Verification items for the finished model (mm, model axes). A direction names the side the tool comes from. Give positions to 0.01 mm unless a question says otherwise; leave off trailing zeros. Order: outer loops, then holes, each group sorted by start corner. A loop starts at its lowest first (then second) coordinate and runs counter-clockwise, first axis right, second up. Notation, with made-up numbers: (71, 73.5) - (100, 73.5) arc R22 cw to (100, 105.5) - close; hole circle Ø1 at (44.5, 6.25). An arc over 180 degrees is marked (long way). Answer as a JSON object with one key per item and string values.
```python
from build123d import *

# Parameters (mm, degrees)
F1_DEPTH = 2
F2_R     = 3
F3_R     = 9
F4_W     = 2
F4_H     = 5
F5_DEPTH = 10
F6_R     = 0.99999


# Not quite as in the source:
# - a fillet or chamfer is up to 0.001 mm smaller than in the source, because OpenCascade refuses the exact size


with BuildPart() as f1:
    # F0 (on Front) → F1 (new body, symmetric)
    with BuildSketch(Plane.XZ):
        Polygon((27.2452607751, 0), (0, 0), (0, -6), (25, -6), (53.6788218176, -46.9576022144), (59.4128861276, -42.94256716), align=None)
    extrude(amount=F1_DEPTH, both=True)

    # F2
    f2_edges = [f1.edges().sort_by_distance(p)[0] for p in [
        (25, 0, -6),
        (53.678822, 0, -46.957602),
        (59.412886, 0, -42.942567),
    ]]
    fillet(f2_edges, radius=F2_R)

    # F3
    f3_edges = [f1.edges().sort_by_distance(p)[0] for p in [
        (27.245261, 0, 0),
    ]]
    fillet(f3_edges, radius=F3_R)

    # F4 (on face) → F5 (cut)
    with BuildSketch(Plane(origin=(0, 0, 0), x_dir=(0, -1, 0), z_dir=(-1, 0, 0))):
        with Locations((0, -3)):
            Rectangle(F4_W, F4_H)
    extrude(amount=-F5_DEPTH, mode=Mode.SUBTRACT)

    # F6 (radius 1 in the source; OpenCascade refuses exactly that, so slightly less here)
    f6_edges = [f1.edges().sort_by_distance(p)[0] for p in [
        (43.750416, -2, -22.03376),
        (26.769245, -2, -0.951335),
        (58.117041, -2, -42.735428),
        (11.370982, -2, 0),
        (56.505829, -2, -44.978111),
        (0, -2, -3),
        (53.894604, -2, -45.73384),
        (11.719149, -2, -6),
        (38.926924, -2, -25.889708),
        (24.823545, -2, -6.338968),
        (43.750416, 2, -22.03376),
        (26.769245, 2, -0.951335),
        (58.117041, 2, -42.735428),
        (11.370982, 2, 0),
        (56.505829, 2, -44.978111),
        (0, 2, -3),
        (53.894604, 2, -45.73384),
        (11.719149, 2, -6),
        (38.926924, 2, -25.889708),
        (24.823545, 2, -6.338968),
    ]]
    fillet(f6_edges, radius=F6_R)


solid = f1.part
```
(1) Section check A-A (x = 8). Record the cut outline in (y, z).
Computed values:
{"outline": "(-2, -5) arc R1 ccw to (-1, -6) - (1, -6) arc R1 ccw to (2, -5) - (2, -1) arc R1 ccw to (1, 0) - (-1, 0) arc R1 ccw to (-2, -1) - close; hole (-1, -5.5) - (1, -5.5) - (1, -0.5) - (-1, -0.5) - close"}
(2) Material ranges on line 1 along Z through (x, y) = (9, -0.45); line 2 along Z through (x, y) = (16, 0.55); line 3 along X through (y, z) = (-0.55, -26.5), recorded low to high. Write a range as [from, to].
Computed values:
{"line 1": "z = [-6, -5.5], [-0.5, 0]", "line 2": "z = [-6, 0]", "line 3": "x = [39.35, 47.1]"}
(3) Release check for a two-part mould opening along Z. For faces 4 (the flat face through (5, 0, -5.5)), 5 (the cylindrical face through (39.343, 1.699, -25.987)), 6 (the flat face through (0, 0, -0.3)), 7 (the flat face through (5, 1, -3)) record: pulls with the +Z half, pulls with the -Z half, needs draft (parallel to the pull), parting line crosses it, or undercut.
Computed values:
{"face 4": "undercut", "face 5": "pulls with the -Z half", "face 6": "needs draft", "face 7": "undercut"}
(4) Access from +Z, -Z, +X, -X, +Y, -Y to the whole of each face (thin tool, end or side, straight path). Record for faces 1 (the flat face through (5, 0, -0.5)), 2 (the cylindrical face through (39.343, -1.699, -25.987)), 3 (the flat face through (12, 0, -6)).
Computed values:
{"face 1": "-X", "face 2": "-Z, -X, -Y", "face 3": "-Z, -X, +Y, -Y"}
(5) Section check B-B (y = 0.4). Record the cut outline in (x, z), then the cut area to 3 significant figures.
Computed values:
{"outline": "(0, -6) - (23.44, -6) arc R3 cw to (25.9, -7.28) - (51.96, -44.5) arc R3 ccw to (56.14, -45.24) - (56.88, -44.72) arc R3 ccw to (57.56, -40.46) - (29.95, -3.6) arc R9 ccw to (22.74, 0) - (0, 0) - (0, -0.5) - (10, -0.5) - (10, -5.5) - (0, -5.5) - close", "area": "420 mm²"}
(6) Gauge pin test, flat ends, axial feed: pin 1 Ø2 at (x, y) = (5.5, 0) entering from -Z; pin 2 Ø1 at (x, y) = (47.5, 1.5) entering from -Z; pin 3 Ø2 at (y, z) = (-1.5, -21.5) entering from +X. Record the tip position at first contact, or that the pin passes through.
Computed values:
{"pin 1": "stops at z = -6", "pin 2": "stops at z = -38.71", "pin 3": "stops at x = 44.04"}
(7) Section check C-C (x = 15). Record the cut outline in (y, z), then the cut area to 3 significant figures.
Computed values:
{"outline": "(-2, -5) arc R1 ccw to (-1, -6) - (1, -6) arc R1 ccw to (2, -5) - (2, -1) arc R1 ccw to (1, 0) - (-1, 0) arc R1 ccw to (-2, -1) - close", "area": "23.1 mm²"}
